from build123d import *

# Parameters (mm, degrees)
SKETCH1_W           = 35.339607518
SKETCH1_H           = 63.5
SKETCH1_R           = 12.7
BOSS_EXTRUDE1_DEPTH = 6.35


with BuildPart() as part:
    # Sketch1 → Boss-Extrude1 (new body)
    with BuildSketch(Plane(origin=(0, 0, 0), x_dir=(0, 0, -1), z_dir=(1, 0, 0))):
        with Locations((0, -13.97)):
            Rectangle(SKETCH1_W, SKETCH1_H)
        Circle(SKETCH1_R, mode=Mode.SUBTRACT)
    extrude(amount=BOSS_EXTRUDE1_DEPTH)


solid = part.part
Work out the finished part from the listing and answer in its coordinate system (mm). Coordinates: 2 decimals unless noted, no trailing zeros. Write each loop counter-clockwise with the first axis right and the second up, starting at its lowest first coordinate (ties: lowest second). Pieces come first, ordered by that corner, then holes. Notation, with made-up numbers: M -20,81.5 L 5,81.5 A31 cw 5,116.5 Z; hole C 60,-2 d3. An arc over 180 degrees is marked long. Answer as CSV lines item,"result". Start each with the question number.
Item 1: Consider L1, parallel to Y at x = 5, z = 0; L2, parallel to Y at x = 1.25, z = -11.5; L3, parallel to Z at x = 5.25, y = 2. Determine where each line is inside the solid, lowest interval first.
Item 2: Determine the mould class of faces 1 (the face through (3, 17.78, 0)), 2 (the face through (3, -14, -17.67)), 3 (the face through (3.13, -12.4, 2.75)) for opening direction Y: released by +Y, released by -Y, zero draft, split by the parting line, or undercut.
Item 3: Section B-B on z = 0 is taken. Write down the section's boundary in (x, y).
Item 4: Section A-A on y = 0 is taken. Write down the section's boundary in (x, z), and give its area (3 significant figures).
Item 5: Section C-C on x = 1.25 is taken. Write down the section's boundary in (y, z).
Checks:
1,L1,"y = -45.72 to -12.7, 12.7 to 17.78"
1,L2,"y = -45.72 to -5.39, 5.39 to 17.78"
1,L3,"z = -17.67 to -12.54, 12.54 to 17.67"
2,face 1,"released by +Y"
2,face 2,"zero draft"
2,face 3,"undercut"
3,outline,"M 0,-45.72 L 6.35,-45.72 L 6.35,-12.7 L 0,-12.7 Z; M 0,12.7 L 6.35,12.7 L 6.35,17.78 L 0,17.78 Z"
4,outline,"M 0,-17.67 L 6.35,-17.67 L 6.35,-12.7 L 0,-12.7 Z; M 0,12.7 L 6.35,12.7 L 6.35,17.67 L 0,17.67 Z"
4,area,"63.1 mm²"
5,outline,"M -45.72,-17.67 L 17.78,-17.67 L 17.78,17.67 L -45.72,17.67 Z; hole C 0,0 d25.4"
